Autodesk Inventor part; units mm, degrees
ref_plane "YZ Plane" through (0, 0, 0) normal (1, 0, 0) x (0, 1, 0)
ref_plane "XZ Plane" through (0, 0, 0) normal (0, 1, 0) x (-1, 0, 0)
ref_plane "XY Plane" through (0, 0, 0) normal (0, 0, 1) x (1, 0, 0)
sketch "Эскиз1" plane through (0, 0, 0) normal (1, 0, 0) x (0, 1, 0)
  line L0 (-9.5, 35) -> (9.5, 35)
  line L1 (9.5, 35) -> (9.5, -35)
  line L2 (9.5, -35) -> (-9.5, -35)
  line L3 (-9.5, -35) -> (-9.5, 35)
  line L4 (-9.5, 35) -> (9.5, -35) construction
  line L5 (9.5, 35) -> (-9.5, -35) construction
  line L6 (0, 35) -> (0, 25)
  circle A0 centre (0, 25) radius 3.25
  line L7 (0, -35) -> (0, -25)
  circle A1 centre (0, -25) radius 3.25
  point P0 (0, 0)
  dimension "d0" = 19
  dimension "d1" = 70
  dimension "d2" = 10
  dimension "d3" = 6.5
  dimension "d4" = 10
  dimension "d5" = 6.5
extrude "Выдавливание1" add sketch "Эскиз1" along normal blind 7.8
sketch "Эскиз2" plane through (0, 0, 0) normal (-1, 0, 0) x (0, 0, 1)
  line L0 (-35, 9.5) -> (35, 9.5)
  line L1 (-14.5, -9.5) -> (14.5, -9.5)
  line L2 (14.5, -9.5) -> (14.5, 9.5)
  line L3 (14.5, 9.5) -> (-14.5, 9.5)
  line L4 (-14.5, 9.5) -> (-14.5, -9.5)
  line L5 (-14.5, -9.5) -> (14.5, 9.5) construction
  line L6 (14.5, -9.5) -> (-14.5, 9.5) construction
  point P0 (0, 0)
  dimension "d8" = 29
extrude "Выдавливание2" add sketch "Эскиз2" along normal blind 11
move faces "Перенос1" translate (0, -0.25, 0) faces at (5.2, -9.5, -4.8333)
move faces "Перенос3" translate (0, -1, 0) faces at (5.2, 9.5, 4.8333)
equation "\"d4\" = d2"
equation "\"d5\" = d3"
properties part number "КВ33.044.202 - Фиксатор каретки" material "Пластик АБС"
Read the model definition and answer for the solid it produces. Units are mm, in the model's axes. A direction names the side the tool comes from. Round coordinates to 2 decimals unless told otherwise and drop trailing zeros. Write each loop counter-clockwise with the first axis right and the second up, starting at its lowest first coordinate (ties: lowest second). Pieces come first, ordered by that corner, then holes. Notation, with made-up numbers: (86, 10.5) - (143, 10.5) arc R9 cw to (143, 26.5) - close; hole circle Ø3 at (-7, 18.5). An arc over 180 degrees is marked (long way). One line per question, with ' | ' between items. Start each with the question number.
1. Section D-D (x = -8) is taken. Determine the outline of the cut face in (y, z), and give its area (3 significant figures).
2. For faces 4 (the face through (0, -9.75, 0)), 5 (the face through (-5, -1, 14.5)), 6 (the face through (0, -3, -22)), determine the directions among +Z, -Z, +X, -X, +Y, -Y from which every point of the face is accessible in a straight line to the end or side of a thin tool.
3. Each of these flat-tipped pins is pushed along its axis until it touches: pin 1 (10 mm diameter, centred on y = -1, z = 20, fed in from -X); pin 2 (3 mm diameter, centred on x = -6.5, y = -5, fed in from +Z); pin 3 (4 mm diameter, centred on y = 0, z = 25, fed in from -X); pin 4 (5.5 mm diameter, centred on x = -6.5, y = 3, fed in from -Z). Where does it stop, or does it pass through?
4. Section C-C (x = 3) is taken. Determine the outline of the cut face in (y, z).
5. Section A-A (y = 0) is taken. Determine the outline of the cut face in (x, z).
6. Find the intervals of material crossed by probe 1 along Z at (x, y) = (3, 0); probe 2 along Y at (x, z) = (2.75, -25); probe 3 along Z at (x, y) = (4.25, -1), in increasing order. Write a range as [from, to].
7. Section B-B (z = -25) is taken. Determine the outline of the cut face in (x, y).
8. For a pull along Z with two mould halves and no side action, classify faces 1 (the face through (3.845, -0.705, -21.827)), 2 (the face through (-11, 0, 0)), 3 (the face through (4, 0, -35)) as +Z half, -Z half, draft (parallel to the pull), parting line (faces both ways), or undercut.
Filled in:
1) outline: (-9.75, -14.5) - (8.5, -14.5) - (8.5, 14.5) - (-9.75, 14.5) - close | area: 529 mm²
2) face 4: +Z, -Z, +X, -X, -Y | face 5: +Z, -X, +Y, -Y | face 6: -Z, -X, +Y, -Y
3) pin 1: x = 0 | pin 2: z = 14.5 | pin 3: through | pin 4: z = -14.5
4) outline: (-9.75, -35) - (8.5, -35) - (8.5, 35) - (-9.75, 35) - close; hole circle Ø6.5 at (0, -25); hole circle Ø6.5 at (0, 25)
5) outline: (-11, -14.5) - (0, -14.5) - (0, -21.75) - (7.8, -21.75) - (7.8, 21.75) - (0, 21.75) - (0, 14.5) - (-11, 14.5) - close; (0, -35) - (7.8, -35) - (7.8, -28.25) - (0, -28.25) - close; (0, 28.25) - (7.8, 28.25) - (7.8, 35) - (0, 35) - close
6) probe 1: [-35, -28.25], [-21.75, 21.75], [28.25, 35] | probe 2: [-9.75, -3.25], [3.25, 8.5] | probe 3: [-35, -28.09], [-21.91, 21.91], [28.09, 35]
7) outline: (0, -9.75) - (7.8, -9.75) - (7.8, -3.25) - (0, -3.25) - close; (0, 3.25) - (7.8, 3.25) - (7.8, 8.5) - (0, 8.5) - close
8) face 1: undercut | face 2: draft | face 3: -Z half
